from build123d import *

# Parameters (mm, degrees)
SALIENTE_EXTRUIR1_DEPTH   = 5
SALIENTE_EXTRUIR1_2_DEPTH = 5
SALIENTE_EXTRUIR1_3_DEPTH = 5
SALIENTE_EXTRUIR1_4_DEPTH = 5
SALIENTE_EXTRUIR1_5_DEPTH = 5
CROQUIS1_W                = 1.882038395
CROQUIS1_H                = 3.311920174
CROQUIS1_W_2              = 1.44614363
CROQUIS1_H_2              = 2.931372224
SALIENTE_EXTRUIR1_6_DEPTH = 5
CROQUIS1_W_3              = 0.976947733
CROQUIS1_H_3              = 1.190080085
SALIENTE_EXTRUIR1_7_DEPTH = 5
SALIENTE_EXTRUIR1_8_DEPTH = 5
CROQUIS1_3_W              = 70
CROQUIS1_3_H              = 30
CROQUIS1_3_W_2            = 1.882038395
CROQUIS1_3_H_2            = 3.311920174
CROQUIS1_3_W_3            = 60
CROQUIS1_3_H_3            = 20
SALIENTE_EXTRUIR2_DEPTH   = 4
CROQUIS3_W                = 65
CROQUIS3_H                = 25
CORTAR_EXTRUIR1_DEPTH     = 3


with BuildPart() as part:
    # Croquis1 → Saliente-Extruir1 (new body)
    with BuildSketch(Plane(origin=(0, 0, 0), x_dir=(1, 0, 0), z_dir=(0, 1, 0))):
        Polygon((-379.943592304, 251.423394178), (-381.088562756, 251.423394178), (-382.133986502, 248.111474004), (-381.133986502, 248.111474004), (-380.795875473, 249.462867756), (-380.240129471, 249.462867756), (-379.943592304, 248.138701402), (-378.943592304, 248.138701402), align=None)
        Polygon((-380.498614386, 250.764925918), (-380.795875473, 249.904754056), (-380.2013533, 249.904754056), align=None, mode=Mode.SUBTRACT)
    extrude(amount=SALIENTE_EXTRUIR1_DEPTH)



with BuildPart() as body_2:
    # Croquis1 → Saliente-Extruir1 2 (new body)
    with BuildSketch(Plane(origin=(0, 0, 0), x_dir=(1, 0, 0), z_dir=(0, 1, 0))):
        Polygon((-378.294984375, 251.111377613), (-378.294984375, 251.423394178), (-376.436891972, 251.423394178), (-376.436891972, 251.111377613), (-377.790927393, 248.551558823), (-376.436891972, 248.551558823), (-376.436891972, 248.138701402), (-378.294984375, 248.138701402), (-378.294984375, 248.551558823), (-376.940948953, 251.111377613), align=None)
    extrude(amount=SALIENTE_EXTRUIR1_2_DEPTH)


with BuildPart() as body_3:
    # Croquis1 → Saliente-Extruir1 3 (new body)
    with BuildSketch(Plane(origin=(0, 0, 0), x_dir=(1, 0, 0), z_dir=(0, 1, 0))):
        Polygon((-362.939380698, 251.300316154), (-361.312091548, 251.300316154), (-361.312091548, 251.039680014), (-362.478498726, 251.039680014), (-362.478498726, 249.871397066), (-361.310931064, 249.871397066), (-361.310931064, 249.584160603), (-362.478498726, 249.584160603), (-362.478498726, 248.428480798), (-361.310931064, 248.428480798), (-361.310931064, 247.98839598), (-362.939380698, 247.98839598), align=None)
    extrude(amount=SALIENTE_EXTRUIR1_3_DEPTH)


with BuildPart() as body_4:
    # Croquis1 → Saliente-Extruir1 4 (new body)
    with BuildSketch(Plane(origin=(0, 0, 0), x_dir=(1, 0, 0), z_dir=(0, 1, 0))):
        Polygon((-360.339718911, 248.428480798), (-360.339718911, 251.300316154), (-360.779331555, 251.300316154), (-360.779331555, 247.98839598), (-358.890625378, 247.98839598), (-358.890625378, 248.428480798), align=None)
    extrude(amount=SALIENTE_EXTRUIR1_4_DEPTH)


with BuildPart() as body_5:
    # Croquis1 → Saliente-Extruir1 5 (new body)
    with BuildSketch(Plane(origin=(0, 0, 0), x_dir=(1, 0, 0), z_dir=(0, 1, 0))):
        Polygon((-348.110575355, 247.98839598), (-346.246917904, 247.98839598), (-346.246917904, 249.462867756), (-346.246917904, 249.871397066), (-347.537142293, 249.871397066), (-347.537142293, 250.764925918), (-346.246917904, 250.764925918), (-346.246917904, 251.300316154), (-348.110575355, 251.300316154), (-348.110575355, 249.462867756), (-346.892030098, 249.462867756), (-346.892030098, 248.428480798), (-348.110575355, 248.428480798), align=None)
    extrude(amount=SALIENTE_EXTRUIR1_5_DEPTH)


with BuildPart() as body_6:
    # Croquis1 → Saliente-Extruir1 6 (new body)
    with BuildSketch(Plane(origin=(0, 0, 0), x_dir=(1, 0, 0), z_dir=(0, 1, 0))):
        with Locations((-342.02217467, 249.644356067)):
            Rectangle(CROQUIS1_W, CROQUIS1_H)
        with Locations((-342.011459779, 249.652215762)):
            Rectangle(CROQUIS1_W_2, CROQUIS1_H_2, mode=Mode.SUBTRACT)
    extrude(amount=SALIENTE_EXTRUIR1_6_DEPTH)


with BuildPart() as body_7:
    # Croquis1 → Saliente-Extruir1 7 (new body)
    with BuildSketch(Plane(origin=(0, 0, 0), x_dir=(1, 0, 0), z_dir=(0, 1, 0))):
        Polygon((-338.977474459, 249.644356067), (-338.977474459, 251.300316154), (-340.583262112, 251.300316154), (-340.583262112, 247.98839598), (-340.190237162, 247.98839598), (-340.190237162, 249.644356067), align=None)
        with Locations((-339.701763296, 250.499794098)):
            Rectangle(CROQUIS1_W_3, CROQUIS1_H_3, mode=Mode.SUBTRACT)
    extrude(amount=SALIENTE_EXTRUIR1_7_DEPTH)


with BuildPart() as body_8:
    # Croquis1 → Saliente-Extruir1 8 (new body)
    with BuildSketch(Plane(origin=(0, 0, 0), x_dir=(1, 0, 0), z_dir=(0, 1, 0))):
        Polygon((-344.28749707, 250.764925918), (-344.28749707, 247.98839598), (-344.670110195, 247.98839598), (-344.670110195, 250.764925918), (-345.558798229, 250.764925918), (-345.558798229, 251.300316154), (-343.379752594, 251.300316154), (-343.379752594, 250.764925918), align=None)
    extrude(amount=SALIENTE_EXTRUIR1_8_DEPTH)


with BuildPart() as part_1:
    add(part.part)

    add(body_2.part)  # Saliente-Extruir2 merges body 2

    add(body_3.part)  # Saliente-Extruir2 merges body 3

    add(body_4.part)  # Saliente-Extruir2 merges body 4

    add(body_5.part)  # Saliente-Extruir2 merges body 5

    add(body_6.part)  # Saliente-Extruir2 merges body 6

    add(body_7.part)  # Saliente-Extruir2 merges body 7

    add(body_8.part)  # Saliente-Extruir2 merges body 8
    # Croquis1_3 → Saliente-Extruir2 (add)
    with BuildSketch(Plane(origin=(0, 0, 0), x_dir=(1, 0, 0), z_dir=(0, 1, 0))):
        with Locations((-362.667441108, 237.173755489)):
            Rectangle(CROQUIS1_3_W, CROQUIS1_3_H)
        Polygon((-338.977474459, 251.300316154), (-340.583262112, 251.300316154), (-340.583262112, 247.98839598), (-340.190237162, 247.98839598), (-340.190237162, 249.644356067), (-338.977474459, 249.644356067), align=None, mode=Mode.SUBTRACT)
        with Locations((-342.02217467, 249.644356067)):
            Rectangle(CROQUIS1_3_W_2, CROQUIS1_3_H_2, mode=Mode.SUBTRACT)
        Polygon((-346.246917904, 247.98839598), (-346.246917904, 249.462867756), (-346.246917904, 249.871397066), (-347.537142293, 249.871397066), (-347.537142293, 250.764925918), (-346.246917904, 250.764925918), (-346.246917904, 251.300316154), (-348.110575355, 251.300316154), (-348.110575355, 249.462867756), (-346.892030098, 249.462867756), (-346.892030098, 248.428480798), (-348.110575355, 248.428480798), (-348.110575355, 247.98839598), align=None, mode=Mode.SUBTRACT)
        Polygon((-360.339718911, 251.300316154), (-360.779331555, 251.300316154), (-360.779331555, 247.98839598), (-358.890625378, 247.98839598), (-358.890625378, 248.428480798), (-360.339718911, 248.428480798), align=None, mode=Mode.SUBTRACT)
        Polygon((-381.088562756, 251.423394178), (-382.133986502, 248.111474004), (-381.133986502, 248.111474004), (-380.795875473, 249.462867756), (-380.240129471, 249.462867756), (-379.943592304, 248.138701402), (-378.943592304, 248.138701402), (-379.943592304, 251.423394178), align=None, mode=Mode.SUBTRACT)
        with Locations((-362.667441108, 237.173755489)):
            Rectangle(CROQUIS1_3_W_3, CROQUIS1_3_H_3, mode=Mode.SUBTRACT)
    extrude(amount=SALIENTE_EXTRUIR2_DEPTH)

    # Croquis3 → Cortar-Extruir1 (cut)
    with BuildSketch(Plane.XZ):
        with Locations((-362.667441108, -237.173755489)):
            Rectangle(CROQUIS3_W, CROQUIS3_H)
    extrude(amount=-CORTAR_EXTRUIR1_DEPTH, mode=Mode.SUBTRACT)


solid = part_1.part
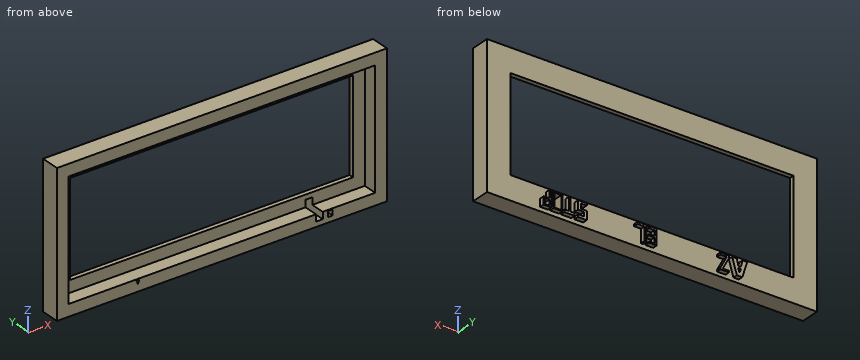
Check sheet for the modelled part. Datum: model origin and axes. Units: mm. Give positions to 0.01 mm unless a question says otherwise; leave off trailing zeros. Order: outer loops, then holes, each group sorted by start corner. A loop starts at its lowest first (then second) coordinate and runs counter-clockwise, first axis right, second up. Notation, with made-up numbers: M -35.5,39 L -3.5,39 A21 cw -3.5,62 Z; hole C 77,82 d2. An arc over 180 degrees is marked long. Answer as CSV lines item,"result". Start each with the question number.
Item 1: Cross-section at A-A on z = -236.75. Enter the section's corners in (x, y).
Item 2: Cross-section at B-B on x = -356. Enter the section's corners in (y, z), plus the area to 3 significant figures.
Item 3: Cross-section at D-D on z = -226. Enter the section's corners in (x, y), plus the area to 3 significant figures.
Item 4: Gauge pin test, flat ends, axial feed: P1, Ø0.5, axis at x = -343.5, y = 4.5, coming from the +Z side; P2, Ø3, axis at x = -368.5, z = -248, coming from the -Y side; P3, Ø0.5, axis at x = -377.5, y = 4.5, coming from the -Z side. Record the tip position at first contact, or that the pin passes through.
Item 5: Thickness scan on line 1 (Z direction, x = -394, y = 2); line 2 (X direction, y = 0.3, z = -243.5); line 3 (Z direction, x = -337.5, y = 3.25). Record the ranges inside material, lowest first. Write a range as [from, to].
Item 6: Cross-section at C-C on y = 1.55. Enter the section's corners in (x, z).
Established:
1,outline,"M -397.67,0 L -395.17,0 L -395.17,3 L -392.67,3 L -392.67,4 L -397.67,4 Z; M -332.67,3 L -330.17,3 L -330.17,0 L -327.67,0 L -327.67,4 L -332.67,4 Z"
2,outline,"M 0,-252.17 L 4,-252.17 L 4,-247.17 L 3,-247.17 L 3,-249.67 L 0,-249.67 Z; M 0,-224.67 L 3,-224.67 L 3,-227.17 L 4,-227.17 L 4,-222.17 L 0,-222.17 Z"
2,area,"25.0 mm^2"
3,outline,"M -397.67,0 L -395.17,0 L -395.17,3 L -330.17,3 L -330.17,0 L -327.67,0 L -327.67,4 L -397.67,4 Z"
3,area,"85.0 mm^2"
4,P1,"stops at z = -250.76"
4,P2,"stops at y = 3"
4,P3,"stops at z = -251.42"
5,line 1,"z = [-252.17, -249.67], [-224.67, -222.17]"
5,line 2,"x = [-397.67, -395.17], [-330.17, -327.67]"
5,line 3,"z = [-252.17, -247.17], [-227.17, -222.17]"
6,outline,"M -397.67,-252.17 L -327.67,-252.17 L -327.67,-222.17 L -397.67,-222.17 Z; hole M -395.17,-249.67 L -342.73,-249.67 L -342.73,-251.12 L -341.29,-251.12 L -341.29,-249.67 L -330.17,-249.67 L -330.17,-224.67 L -395.17,-224.67 Z; hole M -380.8,-249.9 L -380.5,-250.76 L -380.2,-249.9 Z; hole M -340.19,-251.09 L -339.21,-251.09 L -339.21,-249.9 L -340.19,-249.9 Z"
